from build123d import *

# Parameters (mm, degrees)
EXTRUDE_1_DEPTH     = 37.5
SKETCH_2_R          = 3
CUT_EXTRUDE_1_DEPTH = 42.186918984
FILLET_1_R          = 1


with BuildPart() as part:
    # 草图1 → 凸台-拉伸1 (new, symmetric)
    with BuildSketch(Plane.XY):
        with BuildLine():
            Line((-13.74395899, 3.263197464), (-13.74395899, -11.437280558))
            ThreePointArc((-13.74395899, -11.437280558), (-7.74395899, -12.087691895), (-1.74395899, -11.437280558))
            Line((-1.74395899, -11.437280558), (-1.74395899, 3.263197464))
            ThreePointArc((-1.74395899, 3.263197464), (-7.74395899, 1.912308105), (-13.74395899, 3.263197464))
        make_face()
    extrude(amount=EXTRUDE_1_DEPTH, both=True)

    # 草图2 → 切除-拉伸1 (cut, through all)
    with BuildSketch(Plane.ZY.offset(13.74395899)):
        with Locations((30, -4.052061943)):
            Circle(SKETCH_2_R)
        with Locations((-30, -4.052061943)):
            Circle(SKETCH_2_R)
    extrude(amount=-CUT_EXTRUDE_1_DEPTH, mode=Mode.SUBTRACT)

    # 圆角1
    fillet_1_edges = [part.edges().sort_by_distance(p)[0] for p in [
        (-7.74395899, -12.087691895, 37.5),
        (-1.74395899, -4.087041547, 37.5),
        (-1.74395899, -4.052061943, 27),
        (-1.74395899, -4.052061943, -33),
        (-7.74395899, 1.912308105, 37.5),
        (-1.74395899, -4.087041547, -37.5),
        (-7.74395899, -12.087691895, -37.5),
        (-13.74395899, -4.087041547, -37.5),
        (-7.74395899, 1.912308105, -37.5),
        (-13.74395899, -4.087041547, 37.5),
        (-1.74395899, 3.263197464, 0),
        (-1.74395899, -11.437280558, 0),
        (-13.74395899, -11.437280558, 0),
        (-13.74395899, 3.263197464, 0),
    ]]
    fillet(fillet_1_edges, radius=FILLET_1_R)


solid = part.part
Read the model definition and answer for the solid it produces. Units are mm, in the model's axes. Coordinates: 2 decimals unless noted, no trailing zeros. Write each loop counter-clockwise with the first axis right and the second up, starting at its lowest first coordinate (ties: lowest second). Pieces come first, ordered by that corner, then holes. Notation, with made-up numbers: (16, -18) - (32, -18) arc R12 ccw to (32, -7) - close; hole circle Ø1 at (83.5, 5.5). An arc over 180 degrees is marked (long way). One line per question, with ' | ' between items.
Q1. Find section B-B, the plane z = 14.5. Write down the section's boundary in (x, y), plus the area to 3 significant figures.
Result set:
outline: (-13.74, -10.62) arc R1 ccw to (-12.93, -11.6) arc R28 ccw to (-2.56, -11.6) arc R1 ccw to (-1.74, -10.62) - (-1.74, 1.77) arc R1 ccw to (-3.08, 2.71) arc R14 cw to (-12.41, 2.71) arc R1 ccw to (-13.74, 1.77) - close | area: 169 mm^2
Q2. Consider L1, parallel to Z at x = -9.5, y = -4.25; L2, parallel to Z at x = -9.5, y = -3.25; L3, parallel to Y at x = -8.75, z = 29. Determine where each line is inside the solid, lowest interval first. Write a range as [from, to].
Result set:
L1: [-37.5, -32.99], [-27.01, 27.01], [32.99, 37.5] | L2: [-37.5, -32.89], [-27.11, 27.11], [32.89, 37.5] | L3: [-12.07, -6.88], [-1.22, 1.95]
Q3. Determine the mould class of faces 1 (the cylindrical face through (-8, -4, 27)), 2 (the flat face through (-1.744, -5, 1)), 3 (the cylindrical face through (-7.817, -12.088, 0.511)), 4 (the cylindrical face through (-8, -4, -33)) for opening direction Y: +Y half, -Y half, draft (parallel to the pull), parting line (faces both ways), or undercut.
Result set:
face 1: undercut | face 2: draft | face 3: -Y half | face 4: undercut
Q4. Find section A-A, the plane z = 30. Write down the section's boundary in (x, y).
Result set:
outline: (-13.74, -10.62) arc R1 ccw to (-12.93, -11.6) arc R28 ccw to (-2.56, -11.6) arc R1 ccw to (-1.74, -10.62) - (-1.74, -8.05) arc R1 ccw to (-2.74, -7.05) - (-13.74, -7.05) - close; (-13.74, -1.05) - (-2.74, -1.05) arc R1 ccw to (-1.74, -0.05) - (-1.74, 1.77) arc R1 ccw to (-3.08, 2.71) arc R14 cw to (-12.41, 2.71) arc R1 ccw to (-13.74, 1.77) - close
Q5. Find section C-C, the plane x = -10.75. State how many separate pieces and enclosed holes the cut face has, plus the area to 3 significant figures.
Result set:
separate pieces: 1 | enclosed holes: 2 | area: 1,000 mm^2
